from build123d import *

# Parameters (mm, degrees)
ESQUISSE1_R             = 3
ESQUISSE1_R_2           = 2
EXTRUSION1_DEPTH        = 14
CHANFREIN1_SIZE         = 0.25
ENL_V_MAT_EXTRU_1_DEPTH = 10


with BuildPart() as part:
    # Esquisse1 → Extrusion1 (new body)
    with BuildSketch(Plane.XY):
        Circle(ESQUISSE1_R)
        Circle(ESQUISSE1_R_2, mode=Mode.SUBTRACT)
    extrude(amount=EXTRUSION1_DEPTH)

    # Chanfrein1
    chanfrein1_edges = [part.edges().sort_by_distance(p)[0] for p in [
        (-2, 0, 14),
    ]]
    chamfer(chanfrein1_edges, length=CHANFREIN1_SIZE)

    # Esquisse4 → Enlèv. mat.-Extru.1 (cut)
    with BuildSketch(Plane.XY.offset(14)):
        with BuildLine():
            Line((0.25, 2.989565186), (0.25, 0.25))
            Line((0.25, 0.25), (2.989565186, 0.25))
            ThreePointArc((2.989565186, 0.25), (3, 0), (2.989565186, -0.25))
            Line((2.989565186, -0.25), (0.25, -0.25))
            Line((0.25, -0.25), (0.25, -2.989565186))
            ThreePointArc((0.25, -2.989565186), (0, -3), (-0.25, -2.989565186))
            Line((-0.25, -2.989565186), (-0.25, -0.25))
            Line((-0.25, -0.25), (-2.989565186, -0.25))
            ThreePointArc((-2.989565186, -0.25), (-3, 0), (-2.989565186, 0.25))
            Line((-2.989565186, 0.25), (-0.25, 0.25))
            Line((-0.25, 0.25), (-0.25, 2.989565186))
            ThreePointArc((-0.25, 2.989565186), (0, 3), (0.25, 2.989565186))
        make_face()
    extrude(amount=-ENL_V_MAT_EXTRU_1_DEPTH, mode=Mode.SUBTRACT)


solid = part.part
Input: part model. Units: mm. Frame: model coordinates. A direction names the side the tool comes from. Round coordinates to 2 decimals unless told otherwise and drop trailing zeros. Order: outer loops, then holes, each group sorted by start corner. A loop starts at its lowest first (then second) coordinate and runs counter-clockwise, first axis right, second up.
1. Set-up query: faces 4 (the face through (-2.5, -0.25, 9.1)), 5 (the face through (1.49, -1.52, 13.88)), 6 (the face through (1, -2, 0)), 7 (the face through (2, -2, 14)), 8 (the face through (0.25, 2.5, 9.1)). Return all of +Z, -Z, +X, -X, +Y, -Y with unobstructed straight access to the full face (end or side cutting, diameter ignored); none if empty.
The answers:
face 4: +Z, +X, -X
face 5: +Z
face 6: -Z, +X, -X, +Y, -Y
face 7: +Z, +X, -X, +Y, -Y
face 8: +Z, +Y, -Y
2. Cut plane A-A, the plane x = 0. Output: boundary loops of the cut face in (y, z), then the cut area to 3 significant figures.
The answers:
outline: (-3, 0) - (-2, 0) - (-2, 4) - (-3, 4) - close; (2, 0) - (3, 0) - (3, 4) - (2, 4) - close
area: 8.00 mm2
3. Pin query (flat end, axial travel): P1, Ø1.1, axis at x = 2.5, z = 8, coming from the +Y side; P2, Ø1.1, axis at y = 2.5, z = 7, coming from the -X side; P3, Ø1.5, axis at y = -1, z = 3, coming from the +X side. Return the tip coordinate at first contact, or that it passes through.
The answers:
P1: stops at y = 2.28
P2: stops at x = -2.28
P3: stops at x = 2.99
4. Mould query, pull axis Y, two halves, no side actions, for faces 1 (the face through (-1.52, -1.49, 13.88)), 2 (the face through (2.86, 0.9, 6.9)), 3 (the face through (0.25, -2.5, 9.1)). Classes: released by +Y, released by -Y, zero draft, split by the parting line, or undercut.
The answers:
face 1: undercut
face 2: split by the parting line
face 3: zero draft
5. Material intervals for line 1 (X direction, y = 0.6, z = 9.5); line 2 (Y direction, x = 0.8, z = 6); line 3 (X direction, y = -0.9, z = 5), sorted ascending.
The answers:
line 1: x = -2.94 to -1.91, 1.91 to 2.94
line 2: y = -2.89 to -1.83, 1.83 to 2.89
line 3: x = -2.86 to -1.79, 1.79 to 2.86
6. Cut plane C-C, the plane z = 13.25. Output: boundary loops of the cut face in (x, y).
The answers:
outline: (-2.99, -0.25) arc R3 ccw to (-0.25, -2.99) - (-0.25, -1.98) arc R2 cw to (-1.98, -0.25) - close; (-2.99, 0.25) - (-1.98, 0.25) arc R2 cw to (-0.25, 1.98) - (-0.25, 2.99) arc R3 ccw to start; (0.25, -2.99) arc R3 ccw to (2.99, -0.25) - (1.98, -0.25) arc R2 cw to (0.25, -1.98) - close; (0.25, 1.98) arc R2 cw to (1.98, 0.25) - (2.99, 0.25) arc R3 ccw to (0.25, 2.99) - close
7. Cut plane D-D, the plane y = 2.4. Output: boundary loops of the cut face in (x, z), then the cut area to 3 significant figures.
The answers:
outline: (-1.8, 0) - (1.8, 0) - (1.8, 14) - (0.25, 14) - (0.25, 4) - (-0.25, 4) - (-0.25, 14) - (-1.8, 14) - close
area: 45.4 mm2
